Design review of the part shown in the three views and the two pictorial views. Dimensions are in mm from the part's minimum x, y and z. Give positions to 0.01 mm unless a question says otherwise; leave off trailing zeros. Loops run counter-clockwise (first coordinate to the right, second up) from the corner with the lowest first, then second, coordinate; pieces in that order, holes last.
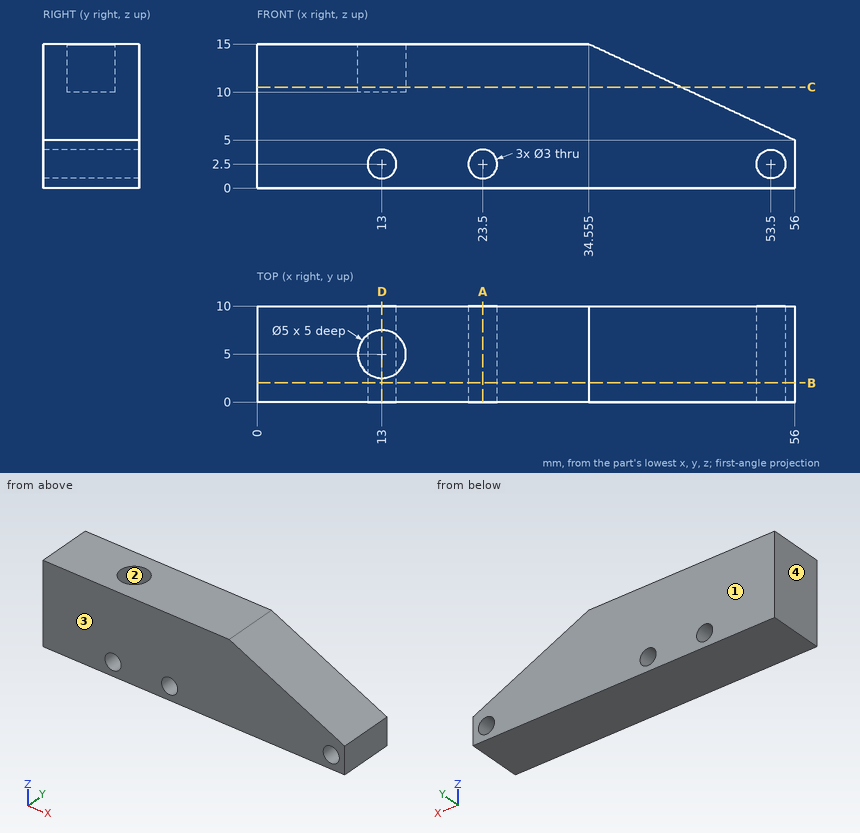
Q1. Draft analysis for pull direction Y (two halves, no side actions). For the marked faces 1, 2, 3 and 4, state which applies: pulls with the +Y half, pulls with the -Y half, needs draft (parallel to the pull), parting line crosses it, or undercut.
Results:
face 1: pulls with the +Y half
face 2: undercut
face 3: pulls with the -Y half
face 4: needs draft
Q2. Take a section at B-B (y = 2). Give the boundary of the cut face in (x, z) (3 decimals).
Results:
outline: (0, 0) - (56, 0) - (56, 5) - (34.555, 15) - (0, 15) - close; hole circle Ø3 at (13, 2.5); hole circle Ø3 at (23.5, 2.5); hole circle Ø3 at (53.5, 2.5)
Q3. Insertion check: pin 1 (2 mm diameter, centred on y = 7.5, z = 6.5, fed in from +X). The pin has a flat end and moves straight along its axis. Give the tip position at first contact, or say it passes through.
Results:
pin 1: stops at x = 54.93
Q4. Take a section at A-A (x = 23.5). Give the boundary of the cut face in (y, z), plus the area to 3 significant figures.
Results:
outline: (0, 0) - (10, 0) - (10, 1) - (0, 1) - close; (0, 4) - (10, 4) - (10, 15) - (0, 15) - close
area: 120 mm2
Q5. Wall thickness on line 1 (Z direction, x = 13, y = 3.5); line 2 (Y direction, x = 13, z = 13.6); line 3 (X direction, y = 7.5, z = 3): over which ranges is each line inside the solid? List them lowest first.
Results:
line 1: z = 0 to 1, 4 to 10
line 2: y = 0 to 2.5, 7.5 to 10
line 3: x = 0 to 11.59, 14.41 to 22.09, 24.91 to 52.09, 54.91 to 56
Q6. Take a section at C-C (z = 10.5). Give the boundary of the cut face in (x, y) (3 decimals).
Results:
outline: (0, 0) - (44.205, 0) - (44.205, 10) - (0, 10) - close; hole circle Ø5 at (13, 5)
Q7. Take a section at D-D (x = 13). Give the boundary of the cut face in (y, z), plus the area to 3 significant figures.
Results:
outline: (0, 0) - (10, 0) - (10, 1) - (0, 1) - close; (0, 4) - (10, 4) - (10, 15) - (7.5, 15) - (7.5, 10) - (2.5, 10) - (2.5, 15) - (0, 15) - close
area: 95.0 mm2
